Design review of the part built by this model. Coordinates are the model's own, in mm. A direction names the side the tool comes from. Coordinates: 2 decimals unless noted, no trailing zeros. Loops run counter-clockwise (first coordinate to the right, second up) from the corner with the lowest first, then second, coordinate; pieces in that order, holes last. Notation, with made-up numbers: (88.25, 31.25) - (105.25, 31.25) arc R28 ccw to (105.25, 67.25) - close; hole circle Ø6 at (25.25, 46). An arc over 180 degrees is marked (long way). Answer in a Markdown table with one row per item. Add a question column.
(1) To check wall thickness, follow L1, parallel to X at y = 3.75, z = 0; L2, parallel to Z at x = 199, y = 5.5; L3, parallel to Z at x = 0, y = 1.5. State the ranges of each line that lie inside material, in increasing order. Write a range as [from, to].
(2) For faces 1 (the face through (-70.07, 3.13, -207.93)), 2 (the face through (91.4, 3.13, 241.22)), 3 (the face through (215.11, 3.13, 43.28)), list the 3-axis set-ups (+Z, -Z, +X, -X, +Y, -Y) from which the entire face can be reached by the end or side of a thin tool; tool diameter is ignored.
(3) We need section C-C, the plane x = 125.5. Write out the cut boundary in (y, z), plus the area to 3 significant figures.
(4) The part is to be moulded in two halves that separate along Z. For faces 4 (the face through (162.557, 3.131, 197.03)), 5 (the face through (-145.036, 3.131, 164.651)), 6 (the face through (89.35, 3.13, -239.29)), say which applies: released by +Z, released by -Z, zero draft, split by the parting line, or undercut.
(5) We need section D-D, the plane z = 263.5. Write out the cut boundary in (x, y), plus the area to 3 significant figures.
(6) We need section B-B, the plane z = -115. Write out the cut boundary in (x, y), plus the area to 3 significant figures.
(7) We need section A-A, the plane y = 2.25. Write out the cut boundary in (x, z).
from build123d import *

# Parameters (mm, degrees)
SKETCH1_R           = 185.399607796
BOSS_EXTRUDE1_DEPTH = 6.35


with BuildPart() as part:
    # Sketch1 → Boss-Extrude1 (new body)
    with BuildSketch(Plane(origin=(0, 0, 0), x_dir=(1, 0, 0), z_dir=(0, 1, 0))):
        with BuildLine():
            Line((-351.324940876, -47.780214023), (-351.324940876, 47.780214023))
            ThreePointArc((-351.324940876, 47.780214023), (-253.254269273, 41.853018609), (-174.699704526, 100.862921435))
            ThreePointArc((-174.699704526, 100.862921435), (-145.322196596, 163.719911973), (-134.05, 232.181410755))
            ThreePointArc((-134.05, 232.181410755), (-69.124504576, 207.712669972), (0, 201.72584287))
            ThreePointArc((0, 201.72584287), (90.381357296, 240.251140111), (134.283591296, 328.146430793))
            Line((134.283591296, 328.146430793), (217.04134958, 280.366216771))
            ThreePointArc((217.04134958, 280.366216771), (162.872911977, 198.398121503), (174.699704526, 100.862921435))
            ThreePointArc((174.699704526, 100.862921435), (214.446701172, 43.992758), (268.1, 0))
            ThreePointArc((268.1, 0), (214.446701172, -43.992758), (174.699704526, -100.862921435))
            ThreePointArc((174.699704526, -100.862921435), (162.872911977, -198.398121503), (217.04134958, -280.366216771))
            Line((217.04134958, -280.366216771), (134.283591296, -328.146430793))
            ThreePointArc((134.283591296, -328.146430793), (90.381357296, -240.251140111), (0, -201.72584287))
            ThreePointArc((0, -201.72584287), (-69.124504576, -207.712669972), (-134.05, -232.181410755))
            ThreePointArc((-134.05, -232.181410755), (-145.322196596, -163.719911973), (-174.699704526, -100.862921435))
            ThreePointArc((-174.699704526, -100.862921435), (-253.254269273, -41.853018609), (-351.324940876, -47.780214023))
        make_face()
        Circle(SKETCH1_R, mode=Mode.SUBTRACT)
    extrude(amount=BOSS_EXTRUDE1_DEPTH)


solid = part.part
Responses:
| question | item | result |
|---|---|---|
| 1 | L1 | x = [-351.32, -185.4], [185.4, 268.1] |
| 1 | L2 | z = [-290.78, -264.58], [-62.34, 62.34], [264.58, 290.78] |
| 1 | L3 | z = [-201.73, -185.4], [185.4, 201.73] |
| 2 | face 1 | -Z, +Y, -Y |
| 2 | face 2 | +Z, +Y, -Y |
| 2 | face 3 | +X, +Y, -Y |
| 3 | outline | (0, -292.36) - (6.35, -292.36) - (6.35, -136.47) - (0, -136.47) - close; (0, 136.47) - (6.35, 136.47) - (6.35, 292.36) - (0, 292.36) - close |
| 3 | area | 1,980 mm2 |
| 4 | face 4 | undercut |
| 4 | face 5 | released by +Z |
| 4 | face 6 | released by -Z |
| 5 | outline | (110.28, 0) - (197.97, 0) - (197.97, 6.35) - (110.28, 6.35) - close |
| 5 | area | 557 mm2 |
| 6 | outline | (-166.19, 0) - (-145.42, 0) - (-145.42, 6.35) - (-166.19, 6.35) - close; (145.42, 0) - (168.41, 0) - (168.41, 6.35) - (145.42, 6.35) - close |
| 6 | area | 278 mm2 |
| 7 | outline | (-351.32, -47.78) arc R142.36 cw to (-174.7, -100.86) arc R254 cw to (-134.05, -232.18) arc R254 cw to (0, -201.73) arc R142.36 cw to (134.28, -328.15) - (217.04, -280.37) arc R142.36 cw to (174.7, -100.86) arc R254 cw to (268.1, 0) arc R254 cw to (174.7, 100.86) arc R142.36 cw to (217.04, 280.37) - (134.28, 328.15) arc R142.36 cw to (0, 201.73) arc R254 cw to (-134.05, 232.18) arc R254 cw to (-174.7, 100.86) arc R142.36 cw to (-351.32, 47.78) - close; hole circle Ø370.8 at (0, 0) |
